Design review of the part built by this model. Coordinates are the model's own, in mm. A direction names the side the tool comes from. Round coordinates to 2 decimals unless told otherwise and drop trailing zeros. Write each loop counter-clockwise with the first axis right and the second up, starting at its lowest first coordinate (ties: lowest second). Pieces come first, ordered by that corner, then holes.
from build123d import *

# Parameters (mm, degrees)
BOSS_EXTRUDE1_DEPTH = 28
BOSS_EXTRUDE2_DEPTH = 28
SKETCH3_R           = 2.55
CUT_EXTRUDE1_DEPTH  = 60.714597447
SKETCH4_R           = 6
CUT_EXTRUDE2_DEPTH  = 28
SKETCH5_W           = 20.4
SKETCH5_H           = 20.4
CUT_EXTRUDE3_DEPTH  = 30
CUT_EXTRUDE4_DEPTH  = 20.4
SKETCH7_R           = 2.6
CUT_EXTRUDE5_DEPTH  = 57.903989341
SKETCH8_R           = 1.5
CUT_EXTRUDE6_DEPTH  = 57.903989341
FILLET2_R           = 3


with BuildPart() as part:
    # Sketch1 → Boss-Extrude1 (new body)
    with BuildSketch(Plane(origin=(0, 0, 0), x_dir=(0, 0, -1), z_dir=(1, 0, 0))):
        Polygon((0, 0), (-24, 0), (-24, -4), (-4, -4), (-4, -24), (0, -24), align=None)
    extrude(amount=BOSS_EXTRUDE1_DEPTH)

    # Sketch2 → Boss-Extrude2 (add)
    with BuildSketch(Plane(origin=(28, 0, 0), x_dir=(0, 0, -1), z_dir=(1, 0, 0))):
        Polygon((2.309401077, -24), (30.582903769, 24.97114317), (6.334192463, 38.97114317), (-16.165807537, 0), (0, 0), (0, -24), align=None)
    extrude(amount=-BOSS_EXTRUDE2_DEPTH)

    # Sketch3 → Cut-Extrude1 (cut, through all)
    with BuildSketch(Plane.XZ.offset(4)):
        with Locations(Location((6.5, 14, 0), (0, 0, 270))):
            Circle(SKETCH3_R)
        with Locations(Location((21.5, 14, 0), (0, 0, 121.860446245))):
            Circle(SKETCH3_R)
    extrude(amount=-CUT_EXTRUDE1_DEPTH, mode=Mode.SUBTRACT)

    # Sketch4 → Cut-Extrude2 (cut)
    with BuildSketch(Plane(origin=(0, 0, 0), x_dir=(1, 0, 0), z_dir=(0, 1, 0))):
        with Locations((6.5, -14)):
            Circle(SKETCH4_R)
        with Locations((21.5, -14)):
            Circle(SKETCH4_R)
    extrude(amount=CUT_EXTRUDE2_DEPTH, mode=Mode.SUBTRACT)

    # Sketch5 → Cut-Extrude3 (cut)
    with BuildSketch(Plane(origin=(0, 31.97114317, -18.458548116), x_dir=(1, 0, 0), z_dir=(0, 0.8660254037844402, -0.49999999999999767))):
        with Locations((14, 0)):
            Rectangle(SKETCH5_W, SKETCH5_H)
    extrude(amount=-CUT_EXTRUDE3_DEPTH, mode=Mode.SUBTRACT)

    # Sketch6 → Cut-Extrude4 (cut)
    with BuildSketch(Plane(origin=(3.8, 0, 0), x_dir=(0, 0, -1), z_dir=(1, 0, 0))):
        Polygon((12.292007234, 0.890381057), (3.458548116, 5.990381057), (3.458548116, -14.409618943), align=None)
    extrude(amount=CUT_EXTRUDE4_DEPTH, mode=Mode.SUBTRACT)

    # Sketch7 → Cut-Extrude5 (cut, through all)
    with BuildSketch(Plane(origin=(28, 0, 0), x_dir=(0, 0, -1), z_dir=(1, 0, 0))):
        with Locations((8.458548116, 14.650635095)):
            Circle(SKETCH7_R)
    extrude(amount=-CUT_EXTRUDE5_DEPTH, mode=Mode.SUBTRACT)

    # Sketch8 → Cut-Extrude6 (cut, through all)
    with BuildSketch(Plane(origin=(28, 0, 0), x_dir=(0, 0, -1), z_dir=(1, 0, 0))):
        with Locations((-4, -4)):
            Circle(SKETCH8_R)
    extrude(amount=-CUT_EXTRUDE6_DEPTH, mode=Mode.SUBTRACT)

    # Fillet2
    fillet2_edges = [part.edges().sort_by_distance(p)[0] for p in [
        (14, -4, 5.5),
        (14, -5.5, 4),
    ]]
    fillet(fillet2_edges, radius=FILLET2_R)


solid = part.part
1) Add section B-B on z = 14. State the section outline as (x, y) points.
2) The part is to be moulded in two halves that separate along Y. For faces 1 (the face through (0, 8, -3)), 2 (the face through (13.86, 24.26, -2.23)), 3 (the face through (14, -4, 16)), say which applies: pulls with the +Y half, pulls with the -Y half, needs draft (parallel to the pull), parting line crosses it, or undercut.
3) Add section D-D on x = 2.25. State the section outline as (y, z) points, and give its area (3 significant figures).
4) For faces 4 (the face through (14.196, -6.146, 3.746)), 5 (the face through (14.2, -3.73, 6.11)), 6 (the face through (24.2, 15.1, -11.2)), list the 3-axis set-ups (+Z, -Z, +X, -X, +Y, -Y) from which the entire face can be reached by the end or side of a thin tool; tool diameter is ignored.
5) For line 1 along X through (y, z) = (-1, 14); line 2 along X through (y, z) = (35, -12); line 3 along Y through (x, z) = (7.25, 3), list the stretches that pass through material, from the lowest coordinate up.
6) For P1, Ø8, axis at x = 23.5, z = 13, coming from the -Y side; P2, Ø1, axis at x = 12, z = -7, coming from the +Y side; P3, Ø8.5, axis at x = 9.5, y = -15.5, coming from the +Z side; P4, Ø5, axis at y = -8.5, z = -17, coming from the -X side, all flat-tipped, find the tip position at first contact; note any pin that passes through.
7) Add section A-A on x = 21.5. State the section outline as (y, z) points.
8) Add section C-C on y = -10. State the section outline as (x, z) points, and give its area (3 significant figures).
Computed:
1. outline: (0, -4) - (3.95, -4) - (3.95, 0) - (0.5, 0) - (0.5, 3.75) - (0, 3.75) - close; (9.05, -4) - (18.95, -4) - (18.95, 0) - (15.5, 0) - (15.5, 3.75) - (12.5, 3.75) - (12.5, 0) - (9.05, 0) - close; (24.05, -4) - (28, -4) - (28, 3.75) - (27.5, 3.75) - (27.5, 0) - (24.05, 0) - close
2. face 1: needs draft
2. face 2: undercut
2. face 3: pulls with the -Y half
3. outline: (-24, -2.31) - (24.97, -30.58) - (38.97, -6.33) - (11.09, 9.76) - (0, 9.76) - (0, 24) - (-4, 24) - (-4, 7.35) arc R3 ccw to (-3, 5.12) arc R1.5 cw (long way) to (-5.12, 3) arc R3 ccw to (-7.35, 4) - (-24, 4) - close; hole circle Ø5.2 at (14.65, -8.46)
3. area: 1,370 mm2
4. face 4: +Z, +X, -X
4. face 5: +X, -X, -Y
4. face 6: none
5. line 1: x = 0 to 3.95, 9.05 to 18.95, 24.05 to 28
5. line 2: x = 0 to 3.8, 24.2 to 28
5. line 3: y = -24 to -5.12, -2.88 to 9.72, 15.2 to 22.8
6. P1: stops at y = -4
6. P2: stops at y = 38.88
6. P3: stops at z = 4
6. P4: passes through
7. outline: (-24, -2.31) - (24.97, -30.58) - (26.87, -27.29) - (-14.41, -3.46) - (5.99, -3.46) - (11.09, 5.37) - (37.07, -9.63) - (38.97, -6.33) - (14.14, 8) - (0, 8) - (0, 11.45) - (-4, 11.45) - (-4, 7.35) arc R3 ccw to (-3, 5.12) arc R1.5 cw (long way) to (-5.12, 3) arc R3 ccw to (-7.35, 4) - (-24, 4) - close; (-4, 16.55) - (0, 16.55) - (0, 24) - (-4, 24) - close
8. outline: (0, -10.39) - (28, -10.39) - (28, 4) - (0, 4) - close; hole (3.8, -6) - (24.2, -6) - (24.2, -3.46) - (3.8, -3.46) - close
8. area: 351 mm2
